Geometry: see drawing. Coordinates: mm, zero at the bounding-box minimum. A direction names the side the tool comes from. Coordinates: 2 decimals unless noted, no trailing zeros. Loops run counter-clockwise (first coordinate to the right, second up) from the corner with the lowest first, then second, coordinate; pieces in that order, holes last. Notation, with made-up numbers: (49, -35) - (65, -35) arc R14 ccw to (65, -15) - close; hole circle Ø10 at (-13, 89). An arc over 180 degrees is marked (long way). Write item = value, one per line. Start each with the question number.
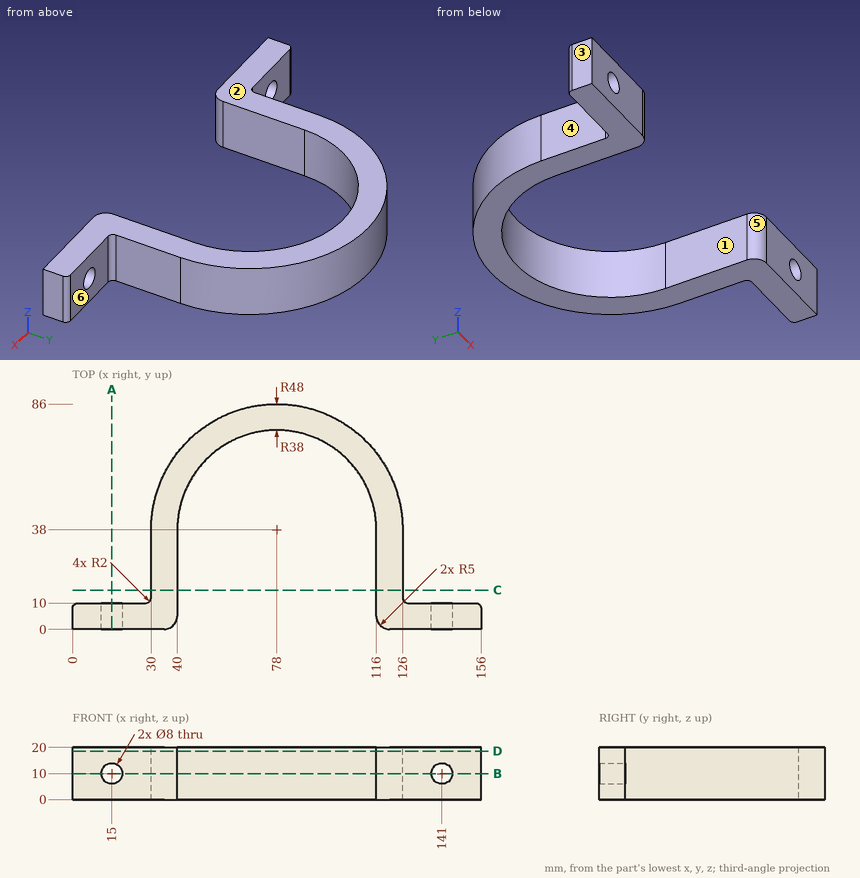
Item 1: Reachability of the marked faces 4, 5 and 6 from +Z, -Z, +X, -X, +Y, -Y: full face, straight path, thin tool, end or side. Return the list, or none.
Item 2: Cut plane D-D (z = 18.5). Return the cut outline in (x, y).
Item 3: Material intervals for L1, parallel to X at y = 4.5, z = 10; L2, parallel to X at y = 7, z = 4.25; L3, parallel to Z at x = 141, y = 2, sorted ascending. Write a range as [from, to].
Item 4: Draft query along X for the marked faces 1, 2 and 3. Return one class per face: released by +X, released by -X, zero draft, split by the parting line, or undercut.
Item 5: First-contact query: pin 1 (6 mm diameter, centred on y = 55, z = 12, fed in from -X); pin 2 (6 mm diameter, centred on y = 24.5, z = 12.5, fed in from +X); pin 3 (1.5 mm diameter, centred on y = 43.5, z = 9, fed in from -X); pin 4 (10 mm diameter, centred on x = 72, y = 66.5, fed in from -Z). Flat tips, straight axial feed; report the tip coordinate or a pass-through.
Item 6: Cut plane B-B (z = 10). Return the cut outline in (x, y), then the cut area to 3 significant figures.
Item 7: Cut plane C-C (y = 15). Return the cut outline in (x, z).
Item 8: Cut plane A-A (x = 15). Return the cut outline in (y, z), then the cut area to 3 significant figures.
Responses:
q1.face_4 = +Z, -Z, -X, +Y
q1.face_5 = +Z, -Z, -Y
q1.face_6 = +Z, -Z, +X, +Y
q2.outline = (0, 0) - (35, 0) arc R5 ccw to (40, 5) - (40, 38) arc R38 cw to (116, 38) - (116, 5) arc R5 ccw to (121, 0) - (156, 0) - (156, 8) arc R2 ccw to (154, 10) - (128, 10) arc R2 cw to (126, 12) - (126, 38) arc R48 ccw to (30, 38) - (30, 12) arc R2 cw to (28, 10) - (2, 10) arc R2 ccw to (0, 8) - close
q3.L1 = [0, 11], [19, 39.97], [116.03, 137], [145, 156]
q3.L2 = [0, 40], [116, 156]
q3.L3 = [0, 6], [14, 20]
q4.face_1 = undercut
q4.face_2 = zero draft
q4.face_3 = released by -X
q5.pin_1 = 32.09
q5.pin_2 = 126
q5.pin_3 = 30.24
q5.pin_4 = through
q6.outline = (0, 0) - (11, 0) - (11, 10) - (2, 10) arc R2 ccw to (0, 8) - close; (19, 0) - (35, 0) arc R5 ccw to (40, 5) - (40, 38) arc R38 cw to (116, 38) - (116, 5) arc R5 ccw to (121, 0) - (137, 0) - (137, 10) - (128, 10) arc R2 cw to (126, 12) - (126, 38) arc R48 ccw to (30, 38) - (30, 12) arc R2 cw to (28, 10) - (19, 10) - close; (145, 0) - (156, 0) - (156, 8) arc R2 ccw to (154, 10) - (145, 10) - close
q6.area = 2,540 mm2
q7.outline = (30, 0) - (40, 0) - (40, 20) - (30, 20) - close; (116, 0) - (126, 0) - (126, 20) - (116, 20) - close
q8.outline = (0, 0) - (10, 0) - (10, 6) - (0, 6) - close; (0, 14) - (10, 14) - (10, 20) - (0, 20) - close
q8.area = 120 mm2
